```python
from build123d import *

# Parameters (mm, degrees)
BOSS_EXTRUDE1_DEPTH = 50.8
SKETCH2_R           = 6.35
SKETCH2_R_2         = 3.175
CUT_EXTRUDE1_DEPTH  = 320.788688435
SKETCH3_W           = 116.84
SKETCH3_H           = 50.8
CUT_EXTRUDE2_DEPTH  = 320.788688435
SKETCH4_W           = 250.150530068
SKETCH4_H           = 117.489254048
CUT_EXTRUDE3_DEPTH  = 244.924275514


with BuildPart() as part:
    # Sketch1 → Boss-Extrude1 (new body)
    with BuildSketch(Plane.XY):
        with BuildLine():
            add(Edge.make_bspline(
                [(0.000560351, 0.000130087), (0.810633127, 7.359196055), (8.649092025, 17.856605174), (26.286719818, 29.975176328), (52.111128271, 42.069215275), (89.597618475, 49.290763054), (131.400792109, 47.884831915), (173.256699242, 40.041104278), (217.961060472, 29.612974894), (256.952064401, 19.528920948), (290.35983767, 8.71099439), (301.273197721, 4.382828139), (314.816918223, -0.516206742), (309.846313895, 0.000130087)],
                knots=[0, 0, 0, 0, 0.060863618, 0.113688265, 0.188608742, 0.312908923, 0.448482434, 0.557612135, 0.691544113, 0.852438279, 0.92975597, 0.976058229, 1, 1, 1, 1], degree=3))
            add(Edge.make_bspline(
                [(309.846313895, 0.000130087), (303.956832565, 1.47095521), (293.989507544, 2.093987313), (276.26402299, 4.514356704), (260.846344817, 5.427413394), (235.858814759, 7.870306192), (205.101424636, 8.838080282), (157.718638092, 9.030650149), (110.497331172, 6.181495223), (66.506197185, -0.586669107), (36.454672816, -6.098499901), (15.316603331, -6.189065841), (1.230714189, -6.924076091), (0.000560351, 0.000130087)],
                knots=[0, 0, 0, 0, 0.057787081, 0.095274891, 0.171021118, 0.205339302, 0.335319146, 0.464904334, 0.658702312, 0.785511947, 0.893517288, 0.94309214, 1, 1, 1, 1], degree=3))
        make_face()
    extrude(amount=BOSS_EXTRUDE1_DEPTH)

    # Sketch2 → Cut-Extrude1 (cut, through all)
    with BuildSketch(Plane.XY.offset(50.8)):
        with Locations((20.32, 10.16)):
            Circle(SKETCH2_R)
        with Locations((227.296313895, 19.050130087)):
            Circle(SKETCH2_R_2)
    extrude(amount=-CUT_EXTRUDE1_DEPTH, mode=Mode.SUBTRACT)

    # Sketch3 → Cut-Extrude2 (cut, through all)
    with BuildSketch(Plane.XY.offset(50.8)):
        with Locations((292.066313895, 19.050130087)):
            Rectangle(SKETCH3_W, SKETCH3_H)
    extrude(amount=-CUT_EXTRUDE2_DEPTH, mode=Mode.SUBTRACT)

    # Sketch4 → Cut-Extrude3 (cut, through all)
    with BuildSketch(Plane.XY.offset(50.8)):
        with Locations((95.871048861, 34.528076629)):
            Rectangle(SKETCH4_W, SKETCH4_H)
    extrude(amount=-CUT_EXTRUDE3_DEPTH, mode=Mode.SUBTRACT)


solid = part.part
```
Check sheet for the modelled part. Datum: model origin and axes. Units: mm. Give positions to 0.01 mm unless a question says otherwise; leave off trailing zeros. Use CSV: the item, a comma, the result in double quotes. Start each with the question number.
Q1. Depth check by flat-ended pin: P1, Ø3, axis at x = 231, z = 19.5, coming from the +Y side; P2, Ø3, axis at x = 227.5, z = 44, coming from the +Y side. Enter the tip coordinate at first touch or a pass-through.
Q2. Scan lines: line 1 along X through (y, z) = (19, 29.5); line 2 along X through (y, z) = (21.5, 28.5); line 3 along Y through (x, z) = (228, 43.5). Record each from-to range of solid material in increasing order.
Q3. Release check for a two-part mould opening along Y. For faces 1 (the cylindrical face through (230.229, 17.834, 25.756)), 2 (the flat face through (225.97, 16, 0)) record: +Y half, -Y half, draft (parallel to the pull), parting line (faces both ways), or undercut.
Working result:
1,P1,"stops at y = 26.52"
1,P2,"stops at y = 27.41"
2,line 1,"x = 220.95 to 224.12, 230.47 to 233.65"
2,line 2,"x = 220.95 to 225.28, 229.32 to 233.65"
2,line 3,"y = 7.98 to 15.95, 22.15 to 26.9"
3,face 1,"undercut"
3,face 2,"draft"
